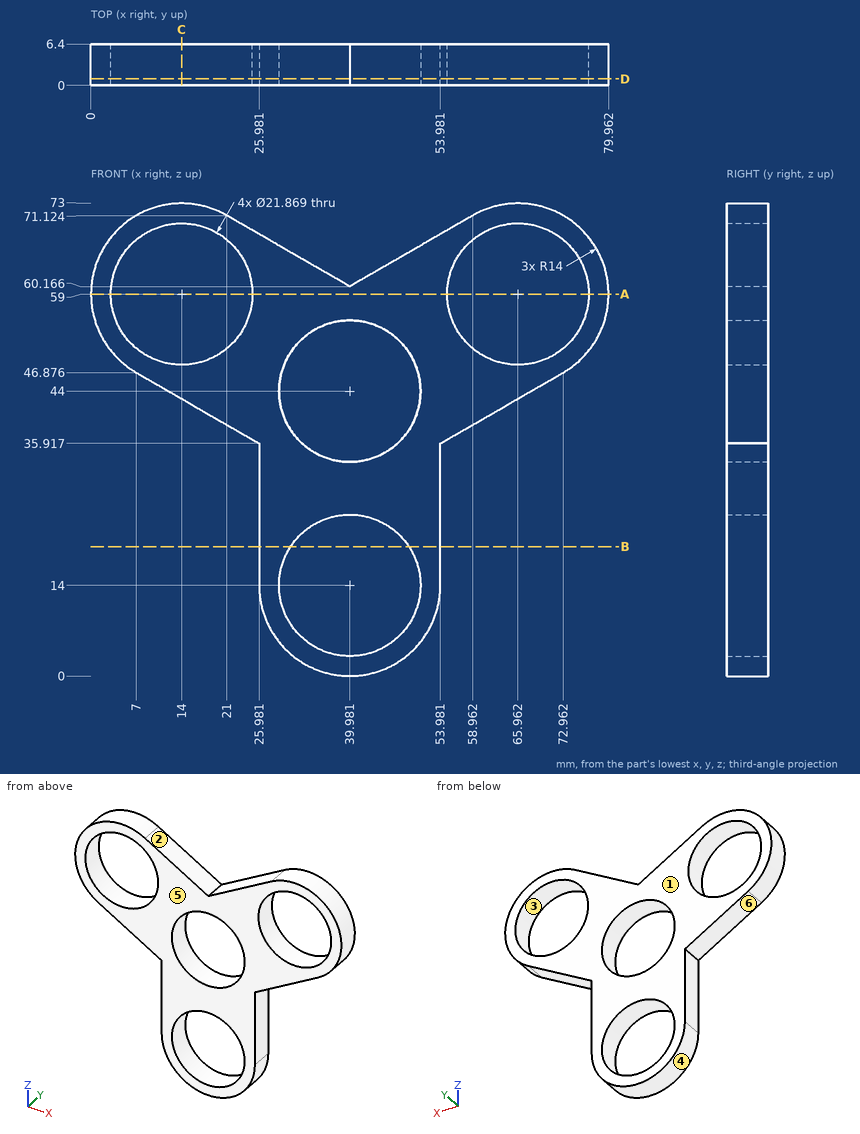
Answer from the drawing. Dimensions are ordinates in mm from the lowest x, y and z of the part. A direction names the side the tool comes from. Round coordinates to 2 decimals unless told otherwise and drop trailing zeros. Write each loop counter-clockwise with the first axis right and the second up, starting at its lowest first coordinate (ties: lowest second). Pieces come first, ordered by that corner, then holes. Notation, with made-up numbers: (26.5, 34.25) -> (46.5, 34.25) arc R21 ccw to (46.5, 53.25) -> close; hole circle Ø7 at (40.25, -28). An arc over 180 degrees is marked (long way). Answer in a Markdown table with one row per item. Add a question column.
1) Find section C-C, the plane x = 14. Determine the outline of the cut face in (y, z) (1 decimal).
2) Find section D-D, the plane y = 1. Determine the outline of the cut face in (x, z) (1 decimal), and give its area (3 significant figures).
3) Given P1, Ø1, axis at y = 2.5, z = 57.5, coming from the +X side; P2, Ø1, axis at y = 5, z = 26, coming from the -X side; P3, Ø1.9, axis at y = 4.5, z = 21, coming from the +X side; P4, Ø10, axis at x = 58.5, z = 34, coming from the -Y side, each flat-ended and moving along its own axis, determine where each tip first touches the part or whether it passes through.
4) Find section A-A, the plane z = 59. Determine the outline of the cut face in (x, y) (1 decimal).
5) Which of the six approach directions +Z, -Z, +X, -X, +Y, -Y give full straight-line access (tool end or side, diameter ignored) to the marked faces 1 and 2?
6) Determine the mould class of the marked faces 3, 4, 5 and 6 for opening direction X: pulls with the +X half, pulls with the -X half, needs draft (parallel to the pull), parting line crosses it, or undercut.
7) Consider line 1 (Z direction, x = 41.5, y = 2) (1 decimal); line 2 (X direction, y = 3.25, z = 52.5) (1 decimal); line 3 (Z direction, x = 42.5, y = 4.75). Determine where each line is inside the solid, lowest interval first.
8) Find section B-B, the plane z = 20. Determine the outline of the cut face in (x, y).
Findings below:
| question | item | result |
|---|---|---|
| 1 | outline | (0, 42.8) -> (6.4, 42.8) -> (6.4, 48.1) -> (0, 48.1) -> close; (0, 69.9) -> (6.4, 69.9) -> (6.4, 73) -> (0, 73) -> close |
| 2 | outline | (7, 46.9) -> (26, 35.9) -> (26, 14) arc R14 ccw to (54, 14) -> (54, 35.9) -> (73, 46.9) arc R14 ccw to (59, 71.1) -> (40, 60.2) -> (21, 71.1) arc R14 ccw to start; hole circle Ø21.9 at (14, 59); hole circle Ø21.9 at (40, 14); hole circle Ø21.9 at (40, 44); hole circle Ø21.9 at (66, 59) |
| 2 | area | 1,600 mm² |
| 3 | P1 | x = 79.93 |
| 3 | P2 | x = 25.98 |
| 3 | P3 | x = 53.98 |
| 3 | P4 | y = 0 |
| 4 | outline | (0, 0) -> (3.1, 0) -> (3.1, 6.4) -> (0, 6.4) -> close; (24.9, 0) -> (55, 0) -> (55, 6.4) -> (24.9, 6.4) -> close; (76.9, 0) -> (80, 0) -> (80, 6.4) -> (76.9, 6.4) -> close |
| 5 | face 1 | +Z, -Z, +X, -X, +Y |
| 5 | face 2 | +Z, +Y, -Y |
| 6 | face 3 | undercut |
| 6 | face 4 | parting line crosses it |
| 6 | face 5 | needs draft |
| 6 | face 6 | pulls with the -X half |
| 7 | line 1 | 0.1 to 3.2, 24.8 to 33.2, 54.8 to 61 |
| 7 | line 2 | 1.6 to 5.2, 22.8 to 33.1, 46.9 to 57.2, 74.8 to 78.4 |
| 7 | line 3 | 0.23 to 3.36, 24.64 to 33.36, 54.64 to 61.62 |
| 8 | outline | (25.98, 0) -> (30.84, 0) -> (30.84, 6.4) -> (25.98, 6.4) -> close; (49.12, 0) -> (53.98, 0) -> (53.98, 6.4) -> (49.12, 6.4) -> close |
